from build123d import *

# Parameters (mm, degrees)
SKETCH1_R           = 4.99
SKETCH1_R_2         = 4.49
BOSS_EXTRUDE1_DEPTH = 5


with BuildPart() as part:
    # Sketch1 → Boss-Extrude1 (new body)
    with BuildSketch(Plane.XY):
        with BuildLine():
            Line((-133.800547442, 2.100285816), (27.342280478, 49.110248457))
            ThreePointArc((27.342280478, 49.110248457), (37.775341878, 45.440970381), (37.648560391, 34.382204707))
            Line((37.648560391, 34.382204707), (8.05154039, -5.913780293))
            ThreePointArc((8.05154039, -5.913780293), (-3.111688569, -9.493023451), (-9.99, 0))
            Line((-9.99, 0), (-8.035082933, 15.898008925))
            ThreePointArc((-8.035082933, 15.898008925), (-9.75887393, 20.317439667), (-14.397978323, 21.308163599))
            Line((-14.397978323, 21.308163599), (-107.124555833, -5.742825892))
            ThreePointArc((-107.124555833, -5.742825892), (-114.923991281, -11.142928518), (-117.92373467, -20.142586361))
            Line((-117.92373467, -20.142586361), (-117.92373467, -53.749229456))
            ThreePointArc((-117.92373467, -53.749229456), (-120.852666858, -60.820297268), (-127.92373467, -63.749229456))
            Line((-127.92373467, -63.749229456), (-131.916457627, -63.749229456))
            ThreePointArc((-131.916457627, -63.749229456), (-137.493140936, -62.674049142), (-142.270365562, -59.602643226))
            Line((-142.270365562, -59.602643226), (-197.550572421, -6.866593112))
            ThreePointArc((-197.550572421, -6.866593112), (-197.866593112, 6.550572421), (-184.449427579, 6.866593112))
            Line((-184.449427579, 6.866593112), (-157.90260529, -18.4584668))
            ThreePointArc((-157.90260529, -18.4584668), (-147.064650772, -20.415954294), (-141, -11.22285762))
            Line((-141, -11.22285762), (-141, -7.499554497))
            ThreePointArc((-141, -7.499554497), (-139.000171074, -1.499782602), (-133.800547442, 2.100285816))
        make_face()
        Circle(SKETCH1_R, mode=Mode.SUBTRACT)
        with Locations((-191, 0)):
            Circle(SKETCH1_R_2, mode=Mode.SUBTRACT)
        with Locations((30, 40)):
            Circle(SKETCH1_R_2, mode=Mode.SUBTRACT)
    extrude(amount=BOSS_EXTRUDE1_DEPTH)


solid = part.part
Here's how the part is built. I have some questions about the finished solid (model axes, mm). A direction names the side the tool comes from. Give positions to 0.01 mm unless a question says otherwise; leave off trailing zeros. Order: outer loops, then holes, each group sorted by start corner. A loop starts at its lowest first (then second) coordinate and runs counter-clockwise, first axis right, second up. Notation, with made-up numbers: (-6.75, -16) -> (52.25, -16) arc R21 cw to (52.25, 11) -> close; hole circle Ø3 at (38.5, 47.5). An arc over 180 degrees is marked (long way). One line per item, written item: value. Start each with the question number.
1. Imagine slicing it at B-B, the plane z = 1.65. List the corners of the cut face in (x, y) for me.
2. For faces 1 (the face through (-195.486, 0.197, 2.465)), 2 (the face through (-117.924, -37, 2)), 3 (the face through (-114.842, -11.035, 2.465)), which set-ups out of +Z, -Z, +X, -X, +Y, -Y let a thin tool reach every point of the face, with its end or its side?
3. I need wall thicknesses on probe 1 along Y at (x, z) = (-0.5, 3.8); probe 2 along Y at (x, z) = (0, 1.7); probe 3 along X at (y, z) = (-47.5, 4). Which ranges of each line are inside material? Lowest first, please. Write a range as from..to.
4. Imagine slicing it at A-A, the plane x = 0. List the corners of the cut face in (y, z) for me, plus the area to 3 significant figures.
5. Will these pins go through, and if not, where does the flat tip stop? pin 1 Ø3 at (x, z) = (-96.5, 1.5) entering from +Y; pin 2 Ø8 at (x, y) = (-191, 0) entering from +Z; pin 3 Ø2 at (x, z) = (-144, 2.5) entering from +Y; pin 4 Ø2 at (y, z) = (-51, 1.5) entering from -X.
6. Imagine slicing it at D-D, the plane x = -113. List the corners of the cut face in (y, z) for me, plus the area to 3 significant figures.
7. Imagine slicing it at C-C, the plane y = 40. List the corners of the cut face in (x, z) for me, plus the area to 3 significant figures.
8. We'd pull the mould along Y, two halves only. Please class faces 4 (the face through (-139.05, -1.57, 2.46)), 5 (the face through (-9.026, 7.838, 2.465)), 6 (the face through (26.437, 37.268, 2.465)), 7 (the face through (-137.419, -62.704, 2.465)): released by +Y, released by -Y, zero draft, split by the parting line, or undercut.
Values follow:
1. outline: (-197.55, -6.87) -> (-142.27, -59.6) arc R15 ccw to (-131.92, -63.75) -> (-127.92, -63.75) arc R10 ccw to (-117.92, -53.75) -> (-117.92, -20.14) arc R15 cw to (-107.12, -5.74) -> (-14.4, 21.31) arc R5 cw to (-8.04, 15.9) -> (-9.99, 0) arc R9.99 ccw to (8.05, -5.91) -> (37.65, 34.38) arc R9.49 ccw to (27.34, 49.11) -> (-133.8, 2.1) arc R10 ccw to (-141, -7.5) -> (-141, -11.22) arc R10 cw to (-157.9, -18.46) -> (-184.45, 6.87) arc R9.49 ccw to start; hole circle Ø8.98 at (-191, 0); hole circle Ø9.98 at (0, 0); hole circle Ø8.98 at (30, 40)
2. face 1: +Z, -Z
2. face 2: +Z, -Z, +X, -Y
2. face 3: +Z, -Z, -Y
3. probe 1: y = -9.98..-4.96, 4.96..40.99
3. probe 2: y = -9.99..-4.99, 4.99..41.13
3. probe 3: x = -154.96..-117.92
4. outline: (-9.99, 0) -> (-4.99, 0) -> (-4.99, 5) -> (-9.99, 5) -> close; (4.99, 0) -> (41.13, 0) -> (41.13, 5) -> (4.99, 5) -> close
4. area: 206 mm2
5. pin 1: stops at y = 13.42
5. pin 2: passes through
5. pin 3: stops at y = -17.22
5. pin 4: stops at x = -152.34
6. outline: (-9.03, 0) -> (8.17, 0) -> (8.17, 5) -> (-9.03, 5) -> close
6. area: 86.0 mm2
7. outline: (-3.89, 0) -> (25.51, 0) -> (25.51, 5) -> (-3.89, 5) -> close; (34.49, 0) -> (39.49, 0) -> (39.49, 5) -> (34.49, 5) -> close
7. area: 172 mm2
8. face 4: released by +Y
8. face 5: undercut
8. face 6: undercut
8. face 7: released by -Y
